```python
from build123d import *

# Parameters (mm, degrees)
SKETCH2_R          = 2
CUT_EXTRUDE1_DEPTH = 34
SKETCH3_W          = 2
SKETCH3_H          = 3.810210747
CUT_EXTRUDE2_DEPTH = 4
CIRPATTERN1_COUNT  = 30
SKETCH4_R          = 35.761747599
CUT_EXTRUDE3_DEPTH = 1.5


with BuildPart() as part:
    # Sketch1 → Revolve1 (revolve)
    with BuildSketch(Plane(origin=(0, 0, 0), x_dir=(0, 0, -1), z_dir=(1, 0, 0))):
        Polygon((-5.5, 0), (-5.5, 26), (-5.400415076, 26), (-4, 24), (0, 24), (0, 0), align=None)
    revolve1 = revolve(axis=Axis((0, 0, 5.5), (0, 0, -1)))

    # Mirror1: Revolve1 across plane
    add(revolve1.mirror(Plane.XY))

    # Sketch2 → Cut-Extrude1 (cut)
    with BuildSketch(Plane.XY.offset(5.5)):
        Circle(SKETCH2_R)
    extrude(amount=-CUT_EXTRUDE1_DEPTH, mode=Mode.SUBTRACT)

    # Sketch3 → Cut-Extrude2 (cut, symmetric)
    with BuildSketch(Plane.XY):
        with Locations((-0.70098694, 25.004508025)):
            Rectangle(SKETCH3_W, SKETCH3_H)
    cut_extrude2 = extrude(amount=CUT_EXTRUDE2_DEPTH, both=True, mode=Mode.SUBTRACT)

    # CirPattern1: Cut-Extrude2 ×30 about axis
    cirpattern1_axis = Axis((0, 0, 0), (0, 0, 1))
    for i in range(1, CIRPATTERN1_COUNT):
        add(cut_extrude2.rotate(cirpattern1_axis, i * 360 / CIRPATTERN1_COUNT), mode=Mode.SUBTRACT)

    # Sketch4 → Cut-Extrude3 (cut)
    with BuildSketch(Plane.XY.offset(5.5)):
        Circle(SKETCH4_R)
    extrude(amount=-CUT_EXTRUDE3_DEPTH, mode=Mode.SUBTRACT)


solid = part.part
```
Geometry: final body of the model. Coordinates: model frame, mm. A direction names the side the tool comes from. Round coordinates to 2 decimals unless told otherwise and drop trailing zeros. Write each loop counter-clockwise with the first axis right and the second up, starting at its lowest first coordinate (ties: lowest second). Pieces come first, ordered by that corner, then holes. Notation, with made-up numbers: (-31.75, -1) -> (25.25, -1) arc R27 ccw to (25.25, 35) -> close; hole circle Ø7 at (-33, 10.5). An arc over 180 degrees is marked (long way). Use CSV: the item, a comma, the result in double quotes. Start each with the question number.
Q1. Reachability of faces 1 (the face through (-17, -16, -4)), 2 (the face through (-1.789, -23.933, 0.056)), 3 (the face through (0, -5, -5.5)), 4 (the face through (-12.62, 20.414, 0.056)), 5 (the face through (1, -23.099, 0)) from +Z, -Z, +X, -X, +Y, -Y: full face, straight path, thin tool, end or side. Return the list, or none.
Q2. First-contact query: pin 1 Ø0.6 at (x, y) = (18, -15.5) entering from +Z; pin 2 Ø5 at (y, z) = (-10.5, -2) entering from +X; pin 3 Ø2 at (x, z) = (-16.5, -1) entering from +Y. Flat tips, straight axial feed; report the tip coordinate or a pass-through.
Q3. Line query: L1, parallel to Y at x = 0, z = 1.25; L2, parallel to Z at x = 22, y = 10; L3, parallel to Y at x = 20, z = 0.75. Output: solid intervals per line, ascending.
Q4. Section A-A (y = 0). Return loops of the section in (x, z), plus the area to 3 significant figures.
Q5. Pull-direction query (X, two-part tool) for faces 6 (the face through (17, 16, -4)), 7 (the face through (6.726, 23.038, 0.056)), 8 (the face through (12.999, 19.108, 0.056)), 9 (the face through (-21.62, -10.42, 0.06)); classes: pulls with the +X half, pulls with the -X half, needs draft (parallel to the pull), parting line crosses it, or undercut.
Result sheet:
1,face 1,"+Z"
1,face 2,"+Z, -X, -Y"
1,face 3,"-Z, +X, -X, +Y, -Y"
1,face 4,"+Z, -X, +Y"
1,face 5,"+Z, -Y"
2,pin 1,"z = -4"
2,pin 2,"x = 22.63"
2,pin 3,"y = 18.32"
3,L1,"-23.1 to -2, 2 to 23.1"
3,L2,"-5.5 to -4.12"
3,L3,"-13.27 to -11.89, -11.56 to 11.56"
4,outline,"(-26, -5.5) -> (-2, -5.5) -> (-2, 4) -> (-24, 4) -> (-24, -4) -> (-26, -5.4) -> close; (2, -5.5) -> (26, -5.5) -> (26, -5.4) -> (24, -4) -> (24, 4) -> (2, 4) -> close"
4,area,"421 mm²"
5,face 6,"undercut"
5,face 7,"pulls with the +X half"
5,face 8,"undercut"
5,face 9,"pulls with the -X half"
